Can you work these out from the model? Positions are in its coordinate system, mm. Face numbers are marked on the shaded views. A direction names the side the tool comes from. Coordinates: 2 decimals unless noted, no trailing zeros. Loops run counter-clockwise (first coordinate to the right, second up) from the corner with the lowest first, then second, coordinate; pieces in that order, holes last.
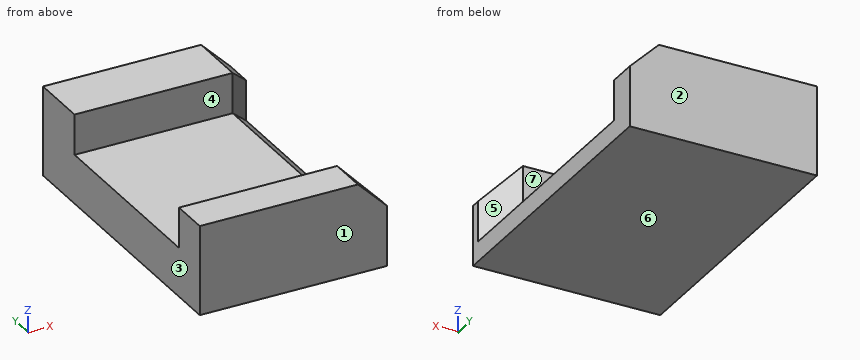
```python
from build123d import *

# Parameters (mm, degrees)
F1_DEPTH = 163.230464
F2_SIZE  = 25.4


with BuildPart() as f1:
    # F0 (on Right) → F1 (new body)
    with BuildSketch(Plane.YZ):
        Polygon((-81.034228, -87.784111), (-81.034228, -52.52336), (-114.317387, -52.52336), (-114.317387, -130.513579), (137.106746, -130.513579), (137.106746, -52.52336), (86.470395, -52.52336), (86.470395, -87.784111), align=None)
    extrude(amount=F1_DEPTH)

    # F2
    f2_edges = [f1.edges().sort_by_distance(p)[0] for p in [
        (163.230464, 2.718084, -87.784111),
        (163.230464, -81.034228, -70.153736),
        (163.230464, 86.470395, -70.153736),
        (163.230464, 111.788571, -52.52336),
        (163.230464, -97.675808, -52.52336),
    ]]
    chamfer(f2_edges, length=F2_SIZE)


solid = f1.part
```
(1) I'm going to push flat-ended pins straight in: pin 1 (1.5 mm diameter, centred on y = -5.5, z = -108.5, fed in from +X); pin 2 (1.5 mm diameter, centred on y = 83, z = -108, fed in from -X); pin 3 (4 mm diameter, centred on x = 87, y = 5.5, fed in from +Z). Where does each tip first touch, or does it pass through?
Check values:
pin 1: stops at x = 159.3
pin 2: stops at x = 0
pin 3: stops at z = -87.78
(2) I want a section at D-D on z = -106.5. Write out the boundary of the cut face in (x, y).
Check values:
outline: (0, -114.32) - (163.23, -114.32) - (163.23, -106.43) - (156.55, -99.75) - (156.55, 105.19) - (163.23, 111.87) - (163.23, 137.11) - (0, 137.11) - close
(3) I want a section at C-C on y = 116.5. Write out the boundary of the cut face in (x, z), then the cut area to 3 significant figures.
Check values:
outline: (0, -130.51) - (163.23, -130.51) - (163.23, -77.92) - (137.83, -52.52) - (0, -52.52) - close
area: 12,400 mm2
(4) If I drill on probe 1 along Y at (x, z) = (125.5, -76); probe 2 along Z at (x, y) = (54, 73); probe 3 along X at (y, z) = (-98.5, -90), over which ranges is the centre line in solid material (lowest first)?
Check values:
probe 1: y = -114.32 to -81.03, 86.47 to 137.11
probe 2: z = -130.51 to -87.78
probe 3: x = 0 to 155.3
(5) Which directions (+Z, -Z, +X, -X, +Y, -Y) give clear straight access to the entire face, cutting with the end or side of a thin tool? Please do the marked faces 5, 6 and 7.
Check values:
face 5: +Z, +X
face 6: -Z, +X, -X, +Y, -Y
face 7: +Z, +X, -X
(6) If we mould it in two halves opening along Y, with no side actions, what happens to the marked faces 1, 2, 3 and 4? For each: released by +Y, released by -Y, zero draft, split by the parting line, or undercut.
Check values:
face 1: released by -Y
face 2: released by +Y
face 3: zero draft
face 4: undercut
(7) I want a section at B-B on z = -66. Write out the boundary of the cut face in (x, y).
Check values:
outline: (0, -114.32) - (151.31, -114.32) - (151.31, -94.51) - (137.83, -81.03) - (0, -81.03) - close; (0, 86.47) - (137.83, 86.47) - (151.31, 99.95) - (151.31, 137.11) - (0, 137.11) - close
(8) I want a section at A-A on x = 130.5. Write out the boundary of the cut face in (y, z), then the cut area to 3 significant figures.
Check values:
outline: (-114.32, -130.51) - (137.11, -130.51) - (137.11, -52.52) - (86.47, -52.52) - (86.47, -87.78) - (-81.03, -87.78) - (-81.03, -52.52) - (-114.32, -52.52) - close
area: 13,700 mm2
